Can you work these out from the model? Positions are in its coordinate system, mm. Face numbers are marked on the shaded views. Round coordinates to 2 decimals unless told otherwise and drop trailing zeros. Order: outer loops, then holes, each group sorted by start corner. A loop starts at its lowest first (then second) coordinate and runs counter-clockwise, first axis right, second up. Notation, with made-up numbers: M 24.5,-5 L 34.5,-5 A9 cw 34.5,9 Z; hole C 72,-39.5 d9. An arc over 180 degrees is marked long. One line per question, with ' | ' between items.
```python
from build123d import *

# Parameters (mm, degrees)
SKETCH2_R           = 15
BOSS_EXTRUDE1_DEPTH = 30
CUT_EXTRUDE1_DEPTH  = 5


with BuildPart() as part:
    # Sketch2 → Boss-Extrude1 (new, symmetric)
    with BuildSketch(Plane.XY):
        Circle(SKETCH2_R)
    extrude(amount=BOSS_EXTRUDE1_DEPTH, both=True)

    # Sketch3 → Cut-Extrude1 (cut)
    with BuildSketch(Plane(origin=(0, 15, 0), x_dir=(1, 0, 0), z_dir=(0, 1, 0))):
        with BuildLine():
            Line((-5, -30), (-5, -10))
            ThreePointArc((-5, -10), (0, -5), (5, -10))
            Line((5, -10), (5, -30))
            ThreePointArc((5, -30), (0, -35), (-5, -30))
        make_face()
    extrude(amount=-CUT_EXTRUDE1_DEPTH, mode=Mode.SUBTRACT)


solid = part.part
```
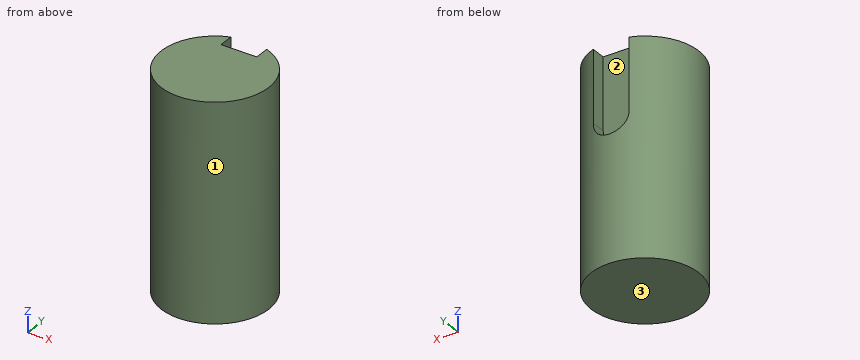
(1) Thinking about a two-plate mould opening in X: for the marked faces 1, 2 and 3, which applies, released by +X, released by -X, zero draft, split by the parting line, or undercut?
Final values:
face 1: split by the parting line | face 2: undercut | face 3: zero draft
(2) If we section it at B-B on x = 0: Please give me the cut outline in (y, z).
Final values:
outline: M -15,-30 L 15,-30 L 15,5 L 10,5 L 10,30 L -15,30 Z
(3) If we section it at D-D on z = 16: Please give me the cut outline in (x, y).
Final values:
outline: M -5,10 L -5,14.14 A15 ccw long 5,14.14 L 5,10 Z
(4) If we section it at A-A on z = -6.5: Please give me the cut outline in (x, y), plus the area to 3 significant figures.
Final values:
outline: C 0,0 d30 | area: 707 mm^2
(5) If we section it at C-C on y = 11.5: Please give me the cut outline in (x, z), plus the area to 3 significant figures.
Final values:
outline: M -9.63,-30 L 9.63,-30 L 9.63,30 L 5,30 L 5,10 A5 cw -5,10 L -5,30 L -9.63,30 Z | area: 916 mm^2
(6) Please list where these lines run through material, in increasing order: probe 1 along Y at (x, z) = (-0.5, 24.5); probe 2 along X at (y, z) = (13.5, 11); probe 3 along X at (y, z) = (4, -6.5). Write a range as [from, to].
Final values:
probe 1: [-14.99, 10] | probe 2: [-6.54, -5], [5, 6.54] | probe 3: [-14.46, 14.46]
(7) Will these pins go through, and if not, where does the flat tip stop? pin 1 Ø4 at (x, z) = (-1, -7.5) entering from -Y; pin 2 Ø4 at (x, z) = (3.5, -22) entering from -Y; pin 3 Ø1.2 at (y, z) = (12, 24.5) entering from -X; pin 4 Ø6 at (x, z) = (11.5, -11.5) entering from -Y.
Final values:
pin 1: y = -15 | pin 2: y = -14.92 | pin 3: x = -9.75 | pin 4: y = -12.36
